```python
from build123d import *

# Parameters (mm, degrees)
SKETCH1_R           = 1.5
SKETCH1_R_2         = 15.5
SKETCH1_R_3         = 1.2
BOSS_EXTRUDE1_DEPTH = 6.35


with BuildPart() as part:
    # Sketch1 → Boss-Extrude1 (new body)
    with BuildSketch(Plane(origin=(0, 0, 0), x_dir=(1, 0, 0), z_dir=(0, 1, 0))):
        with BuildLine():
            Line((0, 0), (38.1, 0))
            Line((38.1, 0), (38.1, 38.1))
            Line((38.1, 38.1), (28.296762992, 61.90754175))
            ThreePointArc((28.296762992, 61.90754175), (19.05, 68.1), (9.803237008, 61.90754175))
            Line((9.803237008, 61.90754175), (0, 38.1))
            Line((0, 38.1), (0, 0))
        make_face()
        with Locations(Location((4.05, 4.05, 0), (0, 0, 270))):
            Circle(SKETCH1_R, mode=Mode.SUBTRACT)
        with Locations(Location((34.05, 4.05, 0), (0, 0, 270))):
            Circle(SKETCH1_R, mode=Mode.SUBTRACT)
        with Locations(Location((34.05, 34.05, 0), (0, 0, 270))):
            Circle(SKETCH1_R, mode=Mode.SUBTRACT)
        with Locations(Location((4.05, 34.05, 0), (0, 0, 270))):
            Circle(SKETCH1_R, mode=Mode.SUBTRACT)
        with Locations(Location((19.05, 19.05, 0), (0, 0, 270))):
            Circle(SKETCH1_R_2, mode=Mode.SUBTRACT)
        with Locations(Location((19.05, 58.1, 0), (0, 0, 270))):
            Circle(SKETCH1_R_3, mode=Mode.SUBTRACT)
    extrude(amount=BOSS_EXTRUDE1_DEPTH)


solid = part.part
```
Read the model definition and answer for the solid it produces. Units are mm, in the model's axes. Give positions to 0.01 mm unless a question says otherwise; leave off trailing zeros. Write each loop counter-clockwise with the first axis right and the second up, starting at its lowest first coordinate (ties: lowest second). Pieces come first, ordered by that corner, then holes. Notation, with made-up numbers: M -23,26.5 L 22,26.5 A18 ccw 22,30.5 Z; hole C 50.5,-29 d6. An arc over 180 degrees is marked long. Put each result on its own line as item: value. Start each with the question number.
1. Consider line 1 along Z through (x, y) = (33, 3.25); line 2 along X through (y, z) = (2.25, -19.05); line 3 along Z through (x, y) = (3.5, 3.25). Determine where each line is inside the solid, lowest interval first.
2. The part is cut by section C-C, the plane y = 4.75. Give the vertices of the cut face in (x, z).
3. This flat-tipped pin is pushed along its axis until it touches: pin 1 Ø1.5 at (x, y) = (29, 5) entering from -Z. Where does it stop, or does it pass through?
4. The part is cut by section D-D, the plane x = 26. Give the vertices of the cut face in (y, z).
5. The part is cut by section A-A, the plane x = 19.05. Give the vertices of the cut face in (y, z).
6. For a pull along X with two mould halves and no side action, classify faces 1 (the flat face through (15, 0, -35)), 2 (the cylindrical face through (5.06, 3.13, -35.16)), 3 (the flat face through (4.97, 3.13, -50.17)) as released by +X, released by -X, zero draft, split by the parting line, or undercut.
7. The part is cut by section B-B, the plane z = -19.05. Give the vertices of the cut face in (x, y).
Final values:
1. line 1: z = -50.49 to -35.12, -32.98 to -25.81, -12.29 to -5.12, -2.98 to 0
1. line 2: x = 0 to 3.55, 34.55 to 38.1
1. line 3: z = -46.6 to -35.45, -32.65 to -5.45, -2.65 to 0
2. outline: M 0,-38.1 L 9.8,-61.91 A10 ccw 28.3,-61.91 L 38.1,-38.1 L 38.1,0 L 0,0 Z; hole C 4.05,-34.05 d3; hole C 4.05,-4.05 d3; hole C 19.05,-19.05 d31; hole C 19.05,-58.1 d2.4; hole C 34.05,-34.05 d3; hole C 34.05,-4.05 d3
3. pin 1: stops at z = -62.02
4. outline: M 0,-65.29 L 6.35,-65.29 L 6.35,-32.9 L 0,-32.9 Z; M 0,-5.2 L 6.35,-5.2 L 6.35,0 L 0,0 Z
5. outline: M 0,-68.1 L 6.35,-68.1 L 6.35,-59.3 L 0,-59.3 Z; M 0,-56.9 L 6.35,-56.9 L 6.35,-34.55 L 0,-34.55 Z; M 0,-3.55 L 6.35,-3.55 L 6.35,0 L 0,0 Z
6. face 1: zero draft
6. face 2: undercut
6. face 3: released by -X
7. outline: M 0,0 L 3.55,0 L 3.55,6.35 L 0,6.35 Z; M 34.55,0 L 38.1,0 L 38.1,6.35 L 34.55,6.35 Z
